Part model, mm, in its own coordinate system. A direction names the side the tool comes from. Round coordinates to 2 decimals unless told otherwise and drop trailing zeros. Write each loop counter-clockwise with the first axis right and the second up, starting at its lowest first coordinate (ties: lowest second). Pieces come first, ordered by that corner, then holes. Notation, with made-up numbers: M 65.25,70 L 90.25,70 A24 cw 90.25,82 Z; hole C 4,43.25 d10. An arc over 180 degrees is marked long. One line per question, with ' | ' between items. Start each with the question number.
1) Drop flat-ended pins along their axis: pin 1 Ø8 at (x, z) = (-3.5, -3) entering from -Y; pin 2 Ø8 at (x, z) = (3, -4.5) entering from +Y; pin 3 Ø5 at (y, z) = (-5, -4) entering from +X; pin 4 Ø3 at (x, z) = (1.5, -6.5) entering from -Y. Give the stop position or say it passes through.
2) Tool access for faces 1 (the face through (0, 5.5, -5)), 2 (the face through (13, 0, -5)), 3 (the face through (-13, 0, -5)): list every direction of +Z, -Z, +X, -X, +Y, -Y with a clear straight run to the whole face (end or side of a thin tool).
3) Saw through at A-A (x = 2). List the corners of the cut face in (y, z), plus the area to 3 significant figures.
4) Wall check: probe 1 along Z at (x, y) = (11.25, 0); probe 2 along Y at (x, z) = (4.75, -8.75); probe 3 along Z at (x, y) = (-11.75, -5.5). Give the ranges that are in metal, low to high. Write a range as [from, to].
5) Saw through at B-B (z = -8). List the corners of the cut face in (x, y), plus the area to 3 significant figures.
```python
from build123d import *

# Parameters (mm, degrees)
EXTRUDE_1_DEPTH = 6
EXTRUDE_2_DEPTH = 10
FILLET_1_R      = 4


with BuildPart() as part:
    # Эскиз1 → Бобышка-Вытянуть1 (new body)
    with BuildSketch(Plane.XY):
        with BuildLine():
            Line((-7.5, 7.5), (7.5, 7.5))
            ThreePointArc((7.5, 7.5), (15, 0), (7.5, -7.5))
            Line((7.5, -7.5), (-7.5, -7.5))
            ThreePointArc((-7.5, -7.5), (-15, 0), (-7.5, 7.5))
        make_face()
    extrude(amount=EXTRUDE_1_DEPTH)

    # Эскиз2 → Бобышка-Вытянуть2 (add)
    with BuildSketch(Plane(origin=(0, 0, 0), x_dir=(-1, 0, 0), z_dir=(0, 0, -1))):
        with BuildLine():
            Line((7.5, 5.5), (-7.5, 5.5))
            ThreePointArc((-7.5, 5.5), (-13, 0), (-7.5, -5.5))
            Line((-7.5, -5.5), (7.5, -5.5))
            ThreePointArc((7.5, -5.5), (13, 0), (7.5, 5.5))
        make_face()
    extrude(amount=EXTRUDE_2_DEPTH)

    # Скругление1
    fillet_1_edges = [part.edges().sort_by_distance(p)[0] for p in [
        (15, 0, 6),
        (0, 7.5, 6),
        (-15, 0, 6),
        (0, -7.5, 6),
    ]]
    fillet(fillet_1_edges, radius=FILLET_1_R)


solid = part.part
```
Answer key:
1) pin 1: stops at y = -7.5 | pin 2: stops at y = 5.5 | pin 3: stops at x = 12.4 | pin 4: stops at y = -5.5
2) face 1: -Z, +X, -X, +Y | face 2: -Z, +X | face 3: -Z, -X
3) outline: M -7.5,0 L -5.5,0 L -5.5,-10 L 5.5,-10 L 5.5,0 L 7.5,0 L 7.5,2 A4 ccw 3.5,6 L -3.5,6 A4 ccw -7.5,2 Z | area: 193 mm2
4) probe 1: z = [-10, 5.99] | probe 2: y = [-5.5, 5.5] | probe 3: z = [0, 4.02]
5) outline: M -7.5,-5.5 L 7.5,-5.5 A5.5 ccw 7.5,5.5 L -7.5,5.5 A5.5 ccw Z | area: 260 mm2
